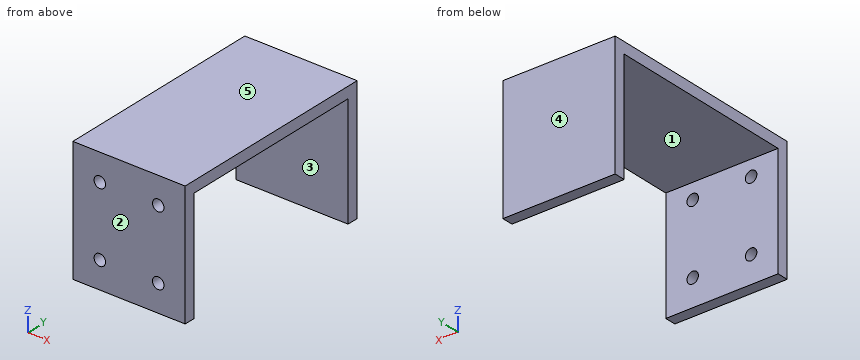
from build123d import *

# Parameters (mm, degrees)
SKETCH_1_W                     = 50
SKETCH_1_H                     = 95.04
EXTRUDE_1_DEPTH                = 5
SKETCH_2_W                     = 50
SKETCH_2_H                     = 5
EXTRUDE_2_DEPTH                = 50
HOLE_START                     = -47.52
HOLE_WIZARD_1_4_20_3_OUTLINE_R = 2.5527
HOLE_WIZARD_1_4_20_3_DEPTH     = 5


# Read off the part's stored shape, not the designer's step: 1/4-20 螺纹孔3
with BuildPart() as part:
    # 草图1 → 凸台-拉伸1 (new body)
    with BuildSketch(Plane.XY):
        Rectangle(SKETCH_1_W, SKETCH_1_H)
    extrude(amount=EXTRUDE_1_DEPTH)

    # 草图2 → 凸台-拉伸2 (add)
    with BuildSketch(Plane(origin=(0, 0, 0), x_dir=(-1, 0, 0), z_dir=(0, 0, -1))):
        with Locations((0, 45.02)):
            Rectangle(SKETCH_2_W, SKETCH_2_H)
        with Locations((0, -45.02)):
            Rectangle(SKETCH_2_W, SKETCH_2_H)
    extrude(amount=EXTRUDE_2_DEPTH)

    # 1/4-20 螺纹孔3 outline → 1/4-20 螺纹孔3 (cut)
    with BuildSketch(Plane(origin=(0, 0, 0), x_dir=(1, 0, 0), z_dir=(0, 1, 0)).offset(HOLE_START)):
        with Locations((13, 7)):
            Circle(HOLE_WIZARD_1_4_20_3_OUTLINE_R)
        with Locations((13, 38)):
            Circle(HOLE_WIZARD_1_4_20_3_OUTLINE_R)
        with Locations((-13, 38)):
            Circle(HOLE_WIZARD_1_4_20_3_OUTLINE_R)
        with Locations((-13, 7)):
            Circle(HOLE_WIZARD_1_4_20_3_OUTLINE_R)
    extrude(amount=HOLE_WIZARD_1_4_20_3_DEPTH, mode=Mode.SUBTRACT)


solid = part.part
Geometry check sheet. Reference: the model listing, model coordinates, mm. Face numbers are marked on the shaded views. A direction names the side the tool comes from. Coordinates: 2 decimals unless noted, no trailing zeros. Order: outer loops, then holes, each group sorted by start corner. A loop starts at its lowest first (then second) coordinate and runs counter-clockwise, first axis right, second up. Notation, with made-up numbers: (25.5, 23) -> (32.5, 23) arc R5 cw to (32.5, 32) -> close; hole circle Ø8 at (39.5, -23.5). An arc over 180 degrees is marked (long way). Use a Markdown table: item, result. Add a question column.
1. Cross-section at B-B (x = -13). Enter the section's corners in (y, z).
2. Set-up check for the marked faces 1 and 2: record each of +Z, -Z, +X, -X, +Y, -Y from which the full face is reachable in a straight line by a thin tool's end or side.
3. Cross-section at A-A (z = -7). Enter the section's corners in (x, y).
4. Cross-section at D-D (x = 5). Enter the section's corners in (y, z), and give its area (3 significant figures).
5. Go/stop test with flat-tipped pins: pin 1 Ø1 at (x, y) = (-5.5, 24) entering from -Z; pin 2 Ø4 at (x, z) = (13, -38) entering from -Y. Record where each tip stops, or that it passes through.
6. Cross-section at C-C (z = -32). Enter the section's corners in (x, y), and give its area (3 significant figures).
7. Material ranges on L1, parallel to Z at x = 13, y = -45; L2, parallel to X at y = -45.25, z = -7; L3, parallel to Y at x = -10, z = -12, recorded low to high.
8. Mould release check, pull along Y, two halves, no side actions. Record for the marked faces 3, 4 and 5: pulls with the +Y half, pulls with the -Y half, needs draft (parallel to the pull), parting line crosses it, or undercut.
Filled sheet:
| question | item | result |
|---|---|---|
| 1 | outline | (-47.52, -50) -> (-42.52, -50) -> (-42.52, -40.55) -> (-47.52, -40.55) -> close; (-47.52, -35.45) -> (-42.52, -35.45) -> (-42.52, -9.55) -> (-47.52, -9.55) -> close; (-47.52, -4.45) -> (-42.52, -4.45) -> (-42.52, 0) -> (42.52, 0) -> (42.52, -50) -> (47.52, -50) -> (47.52, 5) -> (-47.52, 5) -> close |
| 2 | face 1 | -Z, +X, -X |
| 2 | face 2 | +Z, -Z, +X, -X, -Y |
| 3 | outline | (-25, -47.52) -> (-15.55, -47.52) -> (-15.55, -42.52) -> (-25, -42.52) -> close; (-25, 42.52) -> (25, 42.52) -> (25, 47.52) -> (-25, 47.52) -> close; (-10.45, -47.52) -> (10.45, -47.52) -> (10.45, -42.52) -> (-10.45, -42.52) -> close; (15.55, -47.52) -> (25, -47.52) -> (25, -42.52) -> (15.55, -42.52) -> close |
| 4 | outline | (-47.52, -50) -> (-42.52, -50) -> (-42.52, 0) -> (42.52, 0) -> (42.52, -50) -> (47.52, -50) -> (47.52, 5) -> (-47.52, 5) -> close |
| 4 | area | 975 mm2 |
| 5 | pin 1 | z = 0 |
| 5 | pin 2 | y = 42.52 |
| 6 | outline | (-25, -47.52) -> (25, -47.52) -> (25, -42.52) -> (-25, -42.52) -> close; (-25, 42.52) -> (25, 42.52) -> (25, 47.52) -> (-25, 47.52) -> close |
| 6 | area | 500 mm2 |
| 7 | L1 | -50 to -40.55, -35.45 to -9.55, -4.45 to 5 |
| 7 | L2 | -25 to -15.55, -10.45 to 10.45, 15.55 to 25 |
| 7 | L3 | -47.52 to -42.52, 42.52 to 47.52 |
| 8 | face 3 | undercut |
| 8 | face 4 | pulls with the +Y half |
| 8 | face 5 | needs draft |
